Answer from the drawing. Dimensions are ordinates in mm from the lowest x, y and z of the part. A direction names the side the tool comes from. Round coordinates to 2 decimals unless told otherwise and drop trailing zeros. Order: outer loops, then holes, each group sorted by start corner. A loop starts at its lowest first (then second) coordinate and runs counter-clockwise, first axis right, second up. Notation, with made-up numbers: M 31.5,-12 L 73.5,-12 A35 cw 73.5,26 Z; hole C 25,-10 d8. An arc over 180 degrees is marked long. Write item = value, one per line. Start each with the question number.
(1) Each of these flat-tipped pins is pushed along its axis until it touches: pin 1 (2 mm diameter, centred on x = 18.5, z = 3, fed in from -Y); pin 2 (2 mm diameter, centred on y = 18, z = 3.5, fed in from -X) (1 decimal). Where does it stop, or does it pass through?
(2) A cutting plane is placed at A-A, the plane z = 3.05. Determine the outline of the cut face in (x, y) (1 decimal).
(3) Which of the six approach directions +Z, -Z, +X, -X, +Y, -Y give full straight-line access (tool end or side, diameter ignored) to the marked faces 1 and 2?
(4) A cutting plane is placed at C-C, the plane x = 17.5. Determine the outline of the cut face in (y, z).
(5) Straight lines are drawn through the part: probe 1 along Y at (x, z) = (15, 0.55); probe 2 along X at (y, z) = (33, 3.5) (1 decimal); probe 3 along Y at (x, z) = (99, 2.1) (1 decimal). For each, find the intervals that lie inside material, in ascending order. Write a range as from..to.
(6) A cutting plane is placed at B-B, the plane y = 7. Determine the outline of the cut face in (x, z).
(7) A cutting plane is placed at D-D, the plane y = 16. Determine the outline of the cut face in (x, z).
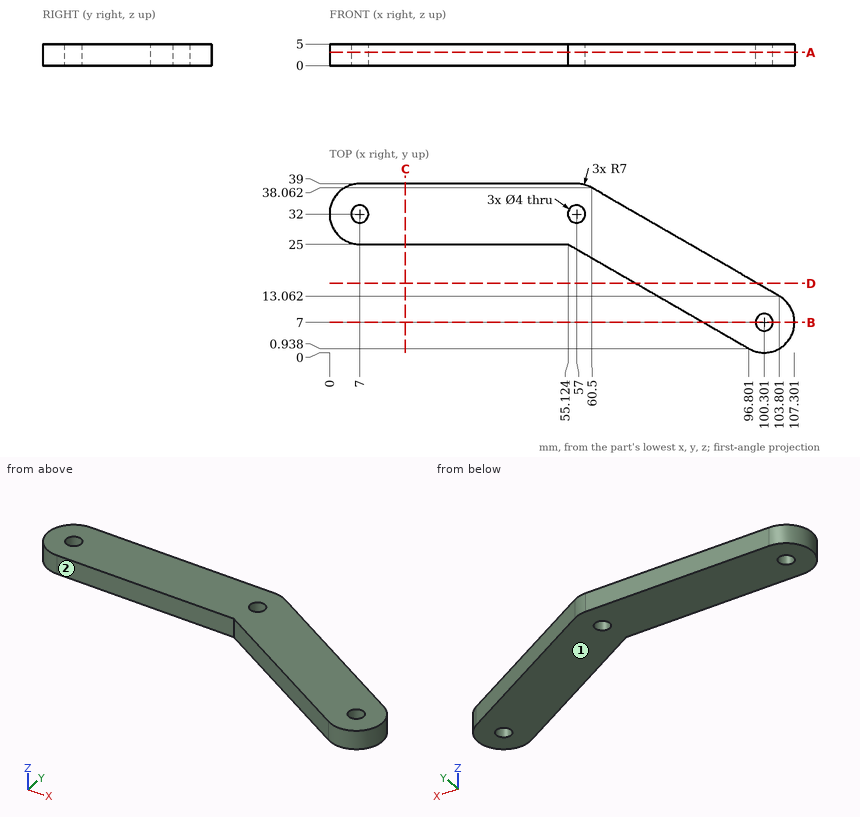
Reported:
q1.pin_1 = 25
q1.pin_2 = 65.5
q2.outline = M 7,25 L 55.1,25 L 96.8,0.9 A7 ccw 103.8,13.1 L 60.5,38.1 A7 ccw 57,39 L 7,39 A7 ccw Z; hole C 7,32 d4; hole C 57,32 d4; hole C 100.3,7 d4
q3.face_1 = -Z, +X, -X, +Y, -Y
q3.face_2 = +Z, -Z, -X, -Y
q4.outline = M 25,0 L 39,0 L 39,5 L 25,5 Z
q5.probe_1 = 25..39
q5.probe_2 = 0.1..5.3, 8.7..55.3, 58.7..69.3
q5.probe_3 = 0.1..5.5, 8.5..15.8
q6.outline = M 86.3,0 L 98.3,0 L 98.3,5 L 86.3,5 Z; M 102.3,0 L 107.3,0 L 107.3,5 L 102.3,5 Z
q7.outline = M 70.71,0 L 98.71,0 L 98.71,5 L 70.71,5 Z
